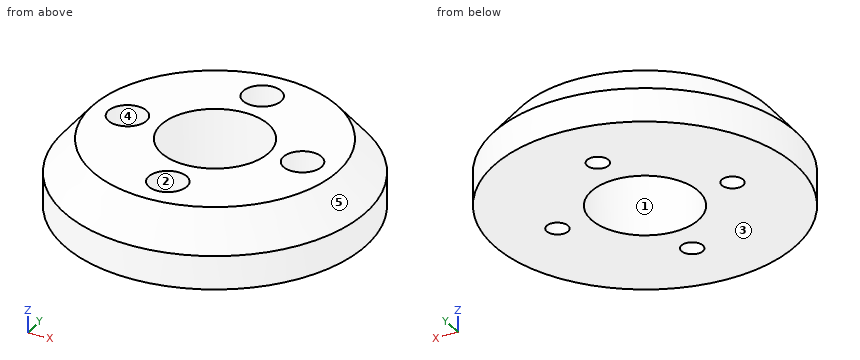
```python
from build123d import *

# Parameters (mm, degrees)
SKETCH1_R               = 22.5
SKETCH1_R_2             = 2.85
BOSS_EXTRUDE1_DEPTH     = 10
SKETCH1_3_R             = 2.85
SKETCH1_3_R_2           = 1.6
BOSS_EXTRUDE2_DEPTH     = 6.5
CHAMFER1_SIZE           = 5
CHAMFER1_SIZE2          = 4.195498156
SKETCH2_R               = 8
CUT_EXTRUDE1_DEPTH      = 1
CUT_EXTRUDE1_DEPTH_BACK = 11


with BuildPart() as part:
    # Sketch1 → Boss-Extrude1 (new body)
    with BuildSketch(Plane(origin=(0, 0, 0), x_dir=(0, 1, 0), z_dir=(0, 0, 1))):
        Circle(SKETCH1_R)
        with Locations((-13, 0)):
            Circle(SKETCH1_R_2, mode=Mode.SUBTRACT)
        with Locations((0, -13)):
            Circle(SKETCH1_R_2, mode=Mode.SUBTRACT)
        with Locations((13, 0)):
            Circle(SKETCH1_R_2, mode=Mode.SUBTRACT)
        with Locations((0, 13)):
            Circle(SKETCH1_R_2, mode=Mode.SUBTRACT)
    extrude(amount=BOSS_EXTRUDE1_DEPTH)

    # Sketch1<3> → Boss-Extrude2 (add)
    with BuildSketch(Plane(origin=(0, 0, 0), x_dir=(0, 1, 0), z_dir=(0, 0, 1))):
        with Locations((-13, 0)):
            Circle(SKETCH1_3_R)
        with Locations((-13, 0)):
            Circle(SKETCH1_3_R_2, mode=Mode.SUBTRACT)
        with Locations((0, 13)):
            Circle(SKETCH1_3_R)
        with Locations((0, 13)):
            Circle(SKETCH1_3_R_2, mode=Mode.SUBTRACT)
        with Locations((13, 0)):
            Circle(SKETCH1_3_R)
        with Locations((13, 0)):
            Circle(SKETCH1_3_R_2, mode=Mode.SUBTRACT)
        with Locations((0, -13)):
            Circle(SKETCH1_3_R)
        with Locations((0, -13)):
            Circle(SKETCH1_3_R_2, mode=Mode.SUBTRACT)
    extrude(amount=BOSS_EXTRUDE2_DEPTH)

    # Chamfer1
    chamfer1_edges = [part.edges().sort_by_distance(p)[0] for p in [
        (0, -22.5, 10),
    ]]
    chamfer1_side = [part.faces().sort_by_distance(p)[0] for p in [
        (0, -22.5, 5),
    ]]
    chamfer(chamfer1_edges, length=CHAMFER1_SIZE, length2=CHAMFER1_SIZE2, reference=chamfer1_side[0])

    # Sketch2 → Cut-Extrude1 (cut, two sides)
    with BuildSketch(Plane.XY.offset(10)) as cut_extrude1_sk:
        Circle(SKETCH2_R)
    extrude(amount=CUT_EXTRUDE1_DEPTH, mode=Mode.SUBTRACT)
    extrude(cut_extrude1_sk.sketch, amount=-CUT_EXTRUDE1_DEPTH_BACK, mode=Mode.SUBTRACT)


solid = part.part
```
Geometry: final body of the model. Coordinates: model frame, mm. Face numbers are marked on the shaded views. A direction names the side the tool comes from. Coordinates: 2 decimals unless noted, no trailing zeros. Order: outer loops, then holes, each group sorted by start corner. A loop starts at its lowest first (then second) coordinate and runs counter-clockwise, first axis right, second up. Notation, with made-up numbers: M 72.25,-12.5 L 118.25,-12.5 A18 ccw 118.25,10.5 Z; hole C -22,83 d8. An arc over 180 degrees is marked long. Answer in a Markdown table with one row per item. Add a question column.
Q1. Contact query for flat-ended pins moving along their axis: P1, Ø1.5, axis at x = 0.5, z = 6, coming from the -Y side; P2, Ø6, axis at y = -15.5, z = 8.5, coming from the -X side; P3, Ø4, axis at x = 0, y = -13, coming from the +Z side; P4, Ø1.7, axis at x = -12.5, y = -0.5, coming from the +Z side. Output: stop coordinate, or through.
Q2. Section query A-A on x = 0. Return the cut outline in (y, z).
Q3. Mould query, pull axis Y, two halves, no side actions, for the marked faces 3, 4 and 5. Classes: released by +Y, released by -Y, zero draft, split by the parting line, or undercut.
Q4. Section query D-D on z = 5.75. Return the cut outline in (x, y), and give its area (3 significant figures).
Q5. Section query C-C on z = 2.5. Return the cut outline in (x, y), and give its area (3 significant figures).
Q6. Reachability of the marked faces 1 and 2 from +Z, -Z, +X, -X, +Y, -Y: full face, straight path, thin tool, end or side. Return the list, or none.
Q7. Line query: L1, parallel to Y at x = 0, z = 2; L2, parallel to Y at x = 0, z = 7.6; L3, parallel to X at y = -2, z = 7. Output: solid intervals per line, ascending.
Completed:
| question | item | result |
|---|---|---|
| 1 | P1 | stops at y = -22.28 |
| 1 | P2 | stops at x = -16.67 |
| 1 | P3 | stops at z = 6.5 |
| 1 | P4 | passes through |
| 2 | outline | M -22.5,0 L -14.6,0 L -14.6,6.5 L -15.85,6.5 L -15.85,10 L -18.3,10 L -22.5,5 Z; M -11.4,0 L -8,0 L -8,10 L -10.15,10 L -10.15,6.5 L -11.4,6.5 Z; M 8,0 L 11.4,0 L 11.4,6.5 L 10.15,6.5 L 10.15,10 L 8,10 Z; M 14.6,0 L 22.5,0 L 22.5,5 L 18.3,10 L 15.85,10 L 15.85,6.5 L 14.6,6.5 Z |
| 3 | face 3 | zero draft |
| 3 | face 4 | undercut |
| 3 | face 5 | split by the parting line |
| 4 | outline | C 0,0 d43.74; hole C -13,0 d3.2; hole C 0,0 d16; hole C 0,-13 d3.2; hole C 0,13 d3.2; hole C 13,0 d3.2 |
| 4 | area | 1,270 mm2 |
| 5 | outline | C 0,0 d45; hole C -13,0 d3.2; hole C 0,0 d16; hole C 0,-13 d3.2; hole C 0,13 d3.2; hole C 13,0 d3.2 |
| 5 | area | 1,360 mm2 |
| 6 | face 1 | +Z, -Z |
| 6 | face 2 | +Z |
| 7 | L1 | y = -22.5 to -14.6, -11.4 to -8, 8 to 11.4, 14.6 to 22.5 |
| 7 | L2 | y = -20.32 to -15.85, -10.15 to -8, 8 to 10.15, 15.85 to 20.32 |
| 7 | L3 | x = -20.73 to -15.03, -10.97 to -7.75, 7.75 to 10.97, 15.03 to 20.73 |
